Print and shaded views of the part. All mm, measured from the part's lowest x, y and z. A direction names the side the tool comes from. Give positions to 0.01 mm unless a question says otherwise; leave off trailing zeros. Write each loop counter-clockwise with the first axis right and the second up, starting at its lowest first coordinate (ties: lowest second). Pieces come first, ordered by that corner, then holes. Notation, with made-up numbers: (23.5, -36) -> (40.5, -36) arc R27 cw to (40.5, -20) -> close; hole circle Ø6 at (88.25, 26). An arc over 180 degrees is marked (long way). Put each result on its own line as item: value.
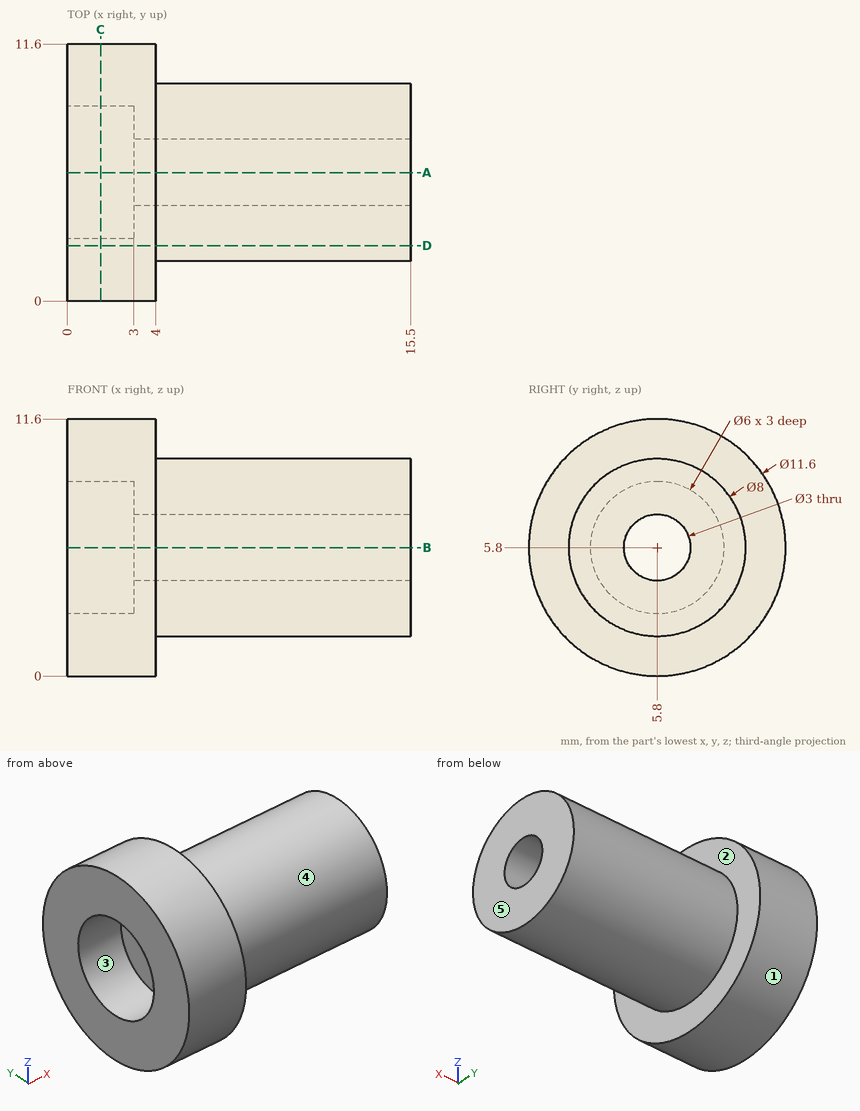
1) Slice it at D-D (y = 2.5). Write the cut outline in (x, z).
Filled sheet:
outline: (0, 1.03) -> (4, 1.03) -> (4, 3.54) -> (15.5, 3.54) -> (15.5, 8.06) -> (4, 8.06) -> (4, 10.57) -> (0, 10.57) -> close
2) Pin check, flat tips, straight feed: pin 1 (3 mm diameter, centred on y = 7, z = 5.5, fed in from -X); pin 2 (3 mm diameter, centred on x = 10, z = 8.5, fed in from +Y); pin 3 (3 mm diameter, centred on x = 8, y = 4, fed in from +Z); pin 4 (2.5 mm diameter, centred on y = 5.8, z = 5.8, fed in from -X). Stop position of each tip, or through.
Filled sheet:
pin 1: x = 3
pin 2: y = 9.62
pin 3: z = 9.79
pin 4: through
3) Wall check: L1, parallel to Y at x = 2.35, z = 5.8; L2, parallel to Y at x = 7, z = 5.8. Give the ranges that are in metal, low to high.
Filled sheet:
L1: 0 to 2.8, 8.8 to 11.6
L2: 1.8 to 4.3, 7.3 to 9.8
4) Tool access for the marked faces 4 and 5: list every direction of +Z, -Z, +X, -X, +Y, -Y with a clear straight run to the whole face (end or side of a thin tool).
Filled sheet:
face 4: +X
face 5: +Z, -Z, +X, +Y, -Y
5) Pull direction Y, two halves, no side cores. Call the marked faces 1, 2 and 3: released by +Y, released by -Y, zero draft, split by the parting line, or undercut.
Filled sheet:
face 1: split by the parting line
face 2: zero draft
face 3: undercut
6) Slice it at A-A (y = 5.8). Write the cut outline in (x, z), plus the area to 3 significant figures.
Filled sheet:
outline: (0, 0) -> (4, 0) -> (4, 1.8) -> (15.5, 1.8) -> (15.5, 4.3) -> (3, 4.3) -> (3, 2.8) -> (0, 2.8) -> close; (0, 8.8) -> (3, 8.8) -> (3, 7.3) -> (15.5, 7.3) -> (15.5, 9.8) -> (4, 9.8) -> (4, 11.6) -> (0, 11.6) -> close
area: 82.9 mm2
7) Slice it at C-C (x = 1.5). Write the cut outline in (y, z).
Filled sheet:
outline: circle Ø11.6 at (5.8, 5.8); hole circle Ø6 at (5.8, 5.8)
